The listing builds one solid part. Answer for the finished solid, in the listing's coordinates (mm). A direction names the side the tool comes from. Give positions to 0.01 mm unless a question says otherwise; leave off trailing zeros. Write each loop counter-clockwise with the first axis right and the second up, starting at its lowest first coordinate (ties: lowest second). Pieces come first, ordered by that corner, then holes. Notation, with made-up numbers: (39, 60.5) - (87, 60.5) arc R19 cw to (87, 78.5) - close; hole circle Ø9 at (14, 72.25). An arc over 180 degrees is marked (long way). One line per question, with ' | ' between items. Start each with the question number.
1. A cutting plane is placed at B-B (x = 30). Determine the outline of the cut face in (y, z), then the cut area to 4 significant figures.
2. A cutting plane is placed at A-A (z = 32). Determine the outline of the cut face in (x, y), then the cut area to 3 significant figures.
3. Given P1, Ø2.5, axis at x = 123.57, z = 46.57, coming from the +Y side, flat-ended and moving along its own axis, determine where the tip first touches the part or whether it passes through.
4. The mould has two halves that part along X. Classify faces 3 (the face through (74.38, 5.07, -0.3)), 4 (the face through (99, 5, 65)), 5 (the face through (0, 5, 25)): +X half, -X half, draft (parallel to the pull), parting line (faces both ways), or undercut.
5. For faces 1 (the face through (30, 5, 4)), 2 (the face through (167.26, 2.46, 1.75)), determine the directions among +Z, -Z, +X, -X, +Y, -Y from which every point of the face is accessible in a straight line to the end or side of a thin tool.
6. A cutting plane is placed at D-D (z = -0.57). Determine the outline of the cut face in (x, y).
7. Find the intervals of material crossed by L1, parallel to X at y = 7, z = 23; L2, parallel to X at y = 2.75, z = 46.57; L3, parallel to Z at x = 77.5, y = 2.75, in increasing order. Write a range as from..to.
8. A cutting plane is placed at C-C (y = 3). State how many separate pieces and enclosed holes the cut face has, then the cut area to 3 significant figures.
Autodesk Inventor part; units mm, degrees
ref_plane "YZ Plane" through (0, 0, 0) normal (1, 0, 0) x (0, 1, 0)
ref_plane "XZ Plane" through (0, 0, 0) normal (0, 1, 0) x (-1, 0, 0)
ref_plane "XY Plane" through (0, 0, 0) normal (0, 0, 1) x (1, 0, 0)
sketch "Sketch1" plane through (0, 0, 0) normal (0, 0, 1) x (1, 0, 0)
  line L0 (0, 0) -> (200, 0)
  line L1 (200, 0) -> (200, 10)
  line L2 (200, 10) -> (0, 10)
  line L3 (0, 10) -> (0, 0)
  dimension "d0" = 200
  dimension "d1" = 10
extrude "Extrusion1" add sketch "Sketch1" along normal blind 70
sketch "Sketch3" plane through (0, 0, 0) normal (0, -1, 0) x (1, 0, 0)
  line L0 (200, 0) -> (200, 70)
  line L1 (200, 38) -> (0, 38)
  line L2 (0, 0) -> (0, 70)
  line L3 (0, 0) -> (200, 0)
  line L4 (200, 20) -> (0, 20)
  line L5 (100, 38) -> (100, 23)
  circle A0 centre (100, 23) radius 15
  circle A1 centre (76.43, -0.57) radius 2.5
  circle A2 centre (76.43, 46.57) radius 2.5
  circle A3 centre (123.57, 46.57) radius 2.5
  circle A4 centre (123.57, -0.57) radius 2.5
  dimension "d11" = 38
  dimension "d12" = 20
  dimension "d13" = 15
  dimension "d14" = 30
  dimension "d15" = 5
  dimension "d16" = 23.57
  dimension "d17" = 23.57
  dimension "d18" = 47.14
  dimension "d19" = 47.14
  dimension "d20" = 5
  dimension "d21" = 5
  dimension "d22" = 5
  dimension "d23" = 47.14
extrude "Extrusion2" cut sketch "Sketch3" against normal blind 10 contours A0 L4 | L4 A0
sketch "Sketch4" plane through (0, 10, 0) normal (0, 1, 0) x (1, 0, 0)
  line L0 (200, 0) -> (200, -70)
  line L1 (200, -23) -> (0, -23)
  line L2 (200, 0) -> (0, 0)
  circle A0 centre (122.5, -23) radius 3
  circle A1 centre (77.5, -23) radius 3
  point P0 (100, -23)
  dimension "d26" = 23
  dimension "d27" = 6
  dimension "d28" = 6
  dimension "d29" = 22.5
  dimension "d30" = 45
sketch "Sketch5" plane through (0, 0, 0) normal (0, 0, -1) x (-1, 0, 0)
  line L0 (-200, 0) -> (-200, 10)
  line L1 (0, 0) -> (-200, 0)
  line L2 (-200, 0) -> (-200, 10)
  line L3 (-200, 10) -> (0, 10)
  line L4 (0, 10) -> (0, 0)
extrude "Extrusion4" add sketch "Sketch5" along normal blind 10
sketch "Sketch6" plane through (0, 10, 70) normal (0, 1, 0) x (1, 0, 0)
  point P0 (0, 70)
sketch "Sketch7" plane through (0, 10, 70) normal (0, 1, 0) x (1, 0, 0)
  line L0 (200, 0) -> (0, 0)
  line L1 (0, 80) -> (0, 0)
  line L2 (200, 0) -> (0, 0)
  line L3 (0, 0) -> (0, 5)
  line L4 (0, 5) -> (200, 5)
  line L5 (200, 5) -> (200, 0)
  point P0 (0, 70)
  dimension "d47" = 5
extrude "Extrusion5" cut sketch "Sketch7" against normal blind 10
sketch "Sketch8" plane through (0, 10, -10) normal (0, 1, 0) x (1, 0, 0)
  line L0 (200, -20) -> (140, -20)
  line L1 (60, -10) -> (140, -10)
  line L2 (60, -20) -> (0, -20)
  point P0 (0, -10)
  point P1 (170, -10)
  point P2 (30, -10)
  point P3 (170, -20)
  point P4 (30, -20)
hole "Hole1" at (30, 10, 0) at (170, 10, 0) direction (0, -1, 0) diameter 6.5 end through all counterbore diameter 11 counterbore depth 5
hole "Hole2" at (77.5, 10, 23) at (122.5, 10, 23) direction (0, -1, 0) diameter 4.917 end through all
sketch "Sketch9" plane through (0, 10, -10) normal (0, 1, 0) x (1, 0, 0)
  point P0 (0, -10)
hole "Hole3" at (123.57, 0, 46.57) at (76.43, 0, 46.57) at (123.57, 0, -0.57) at (76.43, 0, -0.57) direction (0, 1, 0) diameter 4.134 end through all
fillet "Fillet1" radius 5 2 edges at (200, 5, 65) (0, 5, 65)
properties part number "Nap_tren"
Determined:
1) outline: (0, -10) - (10, -10) - (10, -5.5) - (5, -5.5) - (5, -3.25) - (0, -3.25) - close; (0, 3.25) - (5, 3.25) - (5, 5.5) - (10, 5.5) - (10, 65) - (0, 65) - close | area: 662.5 mm2
2) outline: (0, 0) - (88, 0) - (88, 10) - (0, 10) - close; (112, 0) - (200, 0) - (200, 10) - (112, 10) - close | area: 1,760 mm2
3) P1: through
4) face 3: undercut | face 4: draft | face 5: -X half
5) face 1: +Y | face 2: +Y, -Y
6) outline: (0, 0) - (26.8, 0) - (26.8, 5) - (24.53, 5) - (24.53, 10) - (0, 10) - close; (33.2, 0) - (74.36, 0) - (74.36, 10) - (35.47, 10) - (35.47, 5) - (33.2, 5) - close; (78.5, 0) - (121.5, 0) - (121.5, 10) - (78.5, 10) - close; (125.64, 0) - (166.8, 0) - (166.8, 5) - (164.53, 5) - (164.53, 10) - (125.64, 10) - close; (173.2, 0) - (200, 0) - (200, 10) - (175.47, 10) - (175.47, 5) - (173.2, 5) - close
7) L1: 0..75.04, 79.96..85, 115..120.04, 124.96..200 | L2: 0..74.36, 78.5..121.5, 125.64..200 | L3: -10..-2.34, 1.2..20.54, 25.46..44.8, 48.34..65
8) separate pieces: 1 | enclosed holes: 9 | area: 14,100 mm2
